```python
from build123d import *

# Parameters (mm, degrees)
SKETCH1_W           = 500
SKETCH1_H           = 501
BOSS_EXTRUDE1_DEPTH = 6
FILLET1_R           = 44
SKETCH2_W           = 55.5
SKETCH2_H           = 6
CUT_EXTRUDE1_DEPTH  = 10
LPATTERN1_COUNT     = 5
LPATTERN1_PITCH     = 111.2
SKETCH3_W           = 500
SKETCH3_H           = 360
CUT_EXTRUDE2_DEPTH  = 10


with BuildPart() as part:
    # Sketch1 → Boss-Extrude1 (new body)
    with BuildSketch(Plane.XY):
        with Locations((250, 250.5)):
            Rectangle(SKETCH1_W, SKETCH1_H)
    extrude(amount=BOSS_EXTRUDE1_DEPTH)

    # Fillet1
    fillet1_edges = [part.edges().sort_by_distance(p)[0] for p in [
        (0, 501, 3),
        (500, 501, 3),
        (500, 0, 3),
        (0, 0, 3),
    ]]
    fillet(fillet1_edges, radius=FILLET1_R)

    # Sketch2 → Cut-Extrude1 (cut)
    with BuildSketch(Plane(origin=(0, 0, 0), x_dir=(-1, 0, 0), z_dir=(0, 0, -1))):
        with Locations((-27.75, 363)):
            Rectangle(SKETCH2_W, SKETCH2_H)
    cut_extrude1 = extrude(amount=-CUT_EXTRUDE1_DEPTH, mode=Mode.SUBTRACT)

    # LPattern1: Cut-Extrude1 ×5
    with Locations(*[(i * LPATTERN1_PITCH, 0, 0) for i in range(1, LPATTERN1_COUNT)]):
        add(cut_extrude1, mode=Mode.SUBTRACT)

    # Sketch3 → Cut-Extrude2 (cut)
    with BuildSketch(Plane(origin=(0, 0, 0), x_dir=(-1, 0, 0), z_dir=(0, 0, -1))):
        with Locations((-250, 180)):
            Rectangle(SKETCH3_W, SKETCH3_H)
    extrude(amount=-CUT_EXTRUDE2_DEPTH, mode=Mode.SUBTRACT)


solid = part.part
```
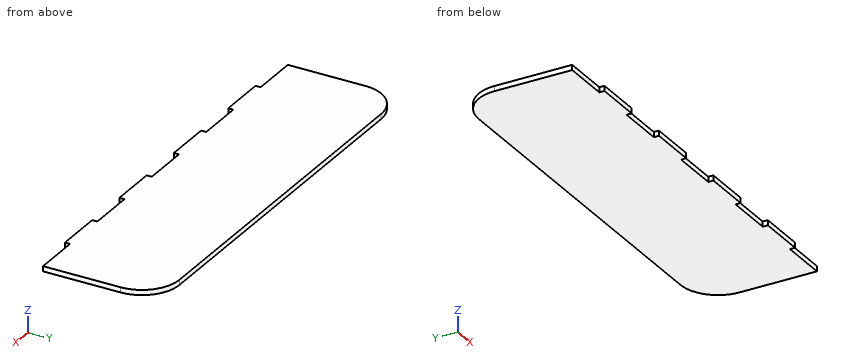
Read the model definition and answer for the solid it produces. Units are mm, in the model's axes. Coordinates: 2 decimals unless noted, no trailing zeros. Write each loop counter-clockwise with the first axis right and the second up, starting at its lowest first coordinate (ties: lowest second). Pieces come first, ordered by that corner, then holes. Notation, with made-up numbers: (-32.75, -15) - (5.25, -15) arc R14 cw to (5.25, 11) - close; hole circle Ø7 at (26, 39). An arc over 180 degrees is marked (long way). Answer as a JSON object with one key per item and string values. Group by question number.
1. Each of these flat-tipped pins is pushed along its axis until it touches: P1, Ø3, axis at x = 21.5, z = 2.5, coming from the -Y side; P2, Ø1.8, axis at y = 362.5, z = 3, coming from the +X side; P3, Ø1.8, axis at y = 362.5, z = 3.5, coming from the -X side. Where does it stop, or does it pass through?
2. A cutting plane is placed at B-B (x = 270.5). Determine the outline of the cut face in (y, z), plus the area to 3 significant figures.
3. A cutting plane is placed at A-A (z = 1.9). Determine the outline of the cut face in (x, y).
4. Consider L1, parallel to Y at x = 361, z = 1.55; L2, parallel to X at y = 486, z = 4.85; L3, parallel to X at y = 478.5, z = 4.1. Determine where each line is inside the solid, lowest interval first. Write a range as [from, to].
Worked out:
{
 "1": {"P1": "stops at y = 366", "P2": "stops at x = 444.8", "P3": "stops at x = 55.5"},
 "2": {"outline": "(366, 0) - (501, 0) - (501, 6) - (366, 6) - close", "area": "810 mm²"},
 "3": {"outline": "(0, 366) - (55.5, 366) - (55.5, 360) - (111.2, 360) - (111.2, 366) - (166.7, 366) - (166.7, 360) - (222.4, 360) - (222.4, 366) - (277.9, 366) - (277.9, 360) - (333.6, 360) - (333.6, 366) - (389.1, 366) - (389.1, 360) - (444.8, 360) - (444.8, 366) - (500, 366) - (500, 457) arc R44 ccw to (456, 501) - (44, 501) arc R44 ccw to (0, 457) - close"},
 "4": {"L1": "y = [366, 501]", "L2": "x = [10.91, 489.09]", "L3": "x = [5.61, 494.39]"}
}
